For this review, take the finished solid that the model builds, in its own axes (mm). Give positions to 0.01 mm unless a question says otherwise; leave off trailing zeros. Write each loop counter-clockwise with the first axis right and the second up, starting at its lowest first coordinate (ties: lowest second). Pieces come first, ordered by that corner, then holes.
1) We need section B-B on z = 4. Give the boundary of the cut face in (x, y), and give its area (3 significant figures).
2) We need section A-A on y = 1.1. Give the boundary of the cut face in (x, z) (3 decimals).
3) Wall thickness on line 1 along Z through (x, y) = (50.8, 0.7); line 2 along X through (y, z) = (1, -35.5); line 3 along Z through (x, y) = (188.5, 1.2): over which ranges is each line inside the solid? List them lowest first.
from build123d import *

# Parameters (mm, degrees)
SKETCH1_R           = 1.0922
BOSS_EXTRUDE1_DEPTH = 1.5875
FILLET1_R           = 6.35


with BuildPart() as part:
    # Sketch1 → Boss-Extrude1 (new body)
    with BuildSketch(Plane(origin=(0, 0, 0), x_dir=(1, 0, 0), z_dir=(0, 1, 0))):
        with BuildLine():
            Line((238.76, 39.37), (0, 39.37))
            ThreePointArc((0, 39.37), (39.37, 0), (0, -39.37))
            Line((0, -39.37), (238.76, -39.37))
            ThreePointArc((238.76, -39.37), (278.13, 0), (238.76, 39.37))
        make_face()
        with Locations((274.955, 0)):
            Circle(SKETCH1_R, mode=Mode.SUBTRACT)
        with Locations((187.96, 36.195)):
            Circle(SKETCH1_R, mode=Mode.SUBTRACT)
        with Locations((50.8, 36.195)):
            Circle(SKETCH1_R, mode=Mode.SUBTRACT)
        with Locations((50.8, -36.195)):
            Circle(SKETCH1_R, mode=Mode.SUBTRACT)
        with Locations((187.96, -36.195)):
            Circle(SKETCH1_R, mode=Mode.SUBTRACT)
    extrude(amount=BOSS_EXTRUDE1_DEPTH)

    # Fillet1
    fillet1_edges = [part.edges().sort_by_distance(p)[0] for p in [
        (0, 0.79375, 39.37),
        (0, 0.79375, -39.37),
    ]]
    fillet(fillet1_edges, radius=FILLET1_R)


solid = part.part
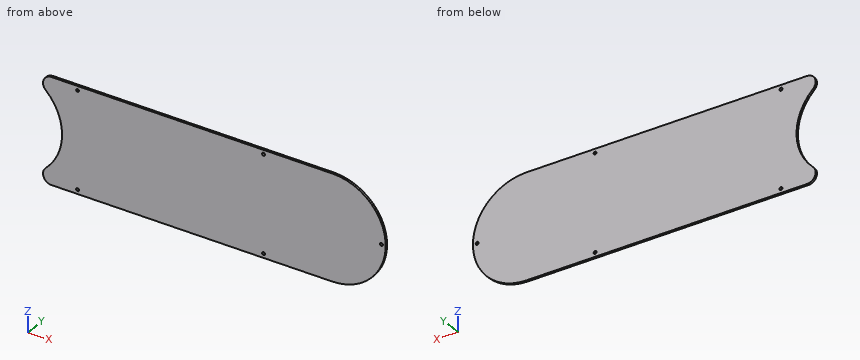
Results list:
1. outline: (39.17, 0) - (277.93, 0) - (277.93, 1.59) - (39.17, 1.59) - close
1. area: 379 mm2
2. outline: (27.231, -28.434) arc R6.35 ccw to (31.623, -39.37) - (238.76, -39.37) arc R39.37 ccw to (238.76, 39.37) - (31.623, 39.37) arc R6.35 ccw to (27.231, 28.434) arc R39.37 cw to start; hole circle Ø2.184 at (50.8, -36.195); hole circle Ø2.184 at (50.8, 36.195); hole circle Ø2.184 at (187.96, -36.195); hole circle Ø2.184 at (187.96, 36.195); hole circle Ø2.184 at (274.955, 0)
3. line 1: z = -39.37 to -37.29, -35.1 to 35.1, 37.29 to 39.37
3. line 2: x = 25.78 to 49.96, 51.64 to 187.12, 188.8 to 255.78
3. line 3: z = -39.37 to -37.14, -35.25 to 35.25, 37.14 to 39.37
